Check sheet for the drawn part. Datum: minimum x, y, z corner. Units: mm. Round coordinates to 2 decimals unless told otherwise and drop trailing zeros. Write each loop counter-clockwise with the first axis right and the second up, starting at its lowest first coordinate (ties: lowest second). Pieces come first, ordered by that corner, then holes. Notation, with made-up numbers: M 64.25,39 L 74.25,39 A7 ccw 74.25,51 Z; hole C -28.5,-3 d10. An arc over 180 degrees is marked long. One line per item, written item: value. Start each with the question number.
Item 1: Section check A-A, the plane x = 2.9. Record the cut outline in (y, z).
Item 2: Section check C-C, the plane y = 2.8. Record the cut outline in (x, z).
Item 3: Thickness scan on probe 1 along Z at (x, y) = (2.7, 0.6); probe 2 along Z at (x, y) = (3.2, 2.7); probe 3 along X at (y, z) = (0.45, 1.65) (1 decimal). Record the ranges inside material, lowest first. Write a range as from..to.
Item 4: Draft check along Z on the marked faces 1, 2 and 3. Enter one of: +Z half, -Z half, draft (parallel to the pull), parting line (faces both ways), or undercut.
Item 5: Section check B-B, the plane z = 1.9. Record the cut outline in (x, y).
Item 6: Section check D-D, the plane x = 1. Record the cut outline in (y, z).
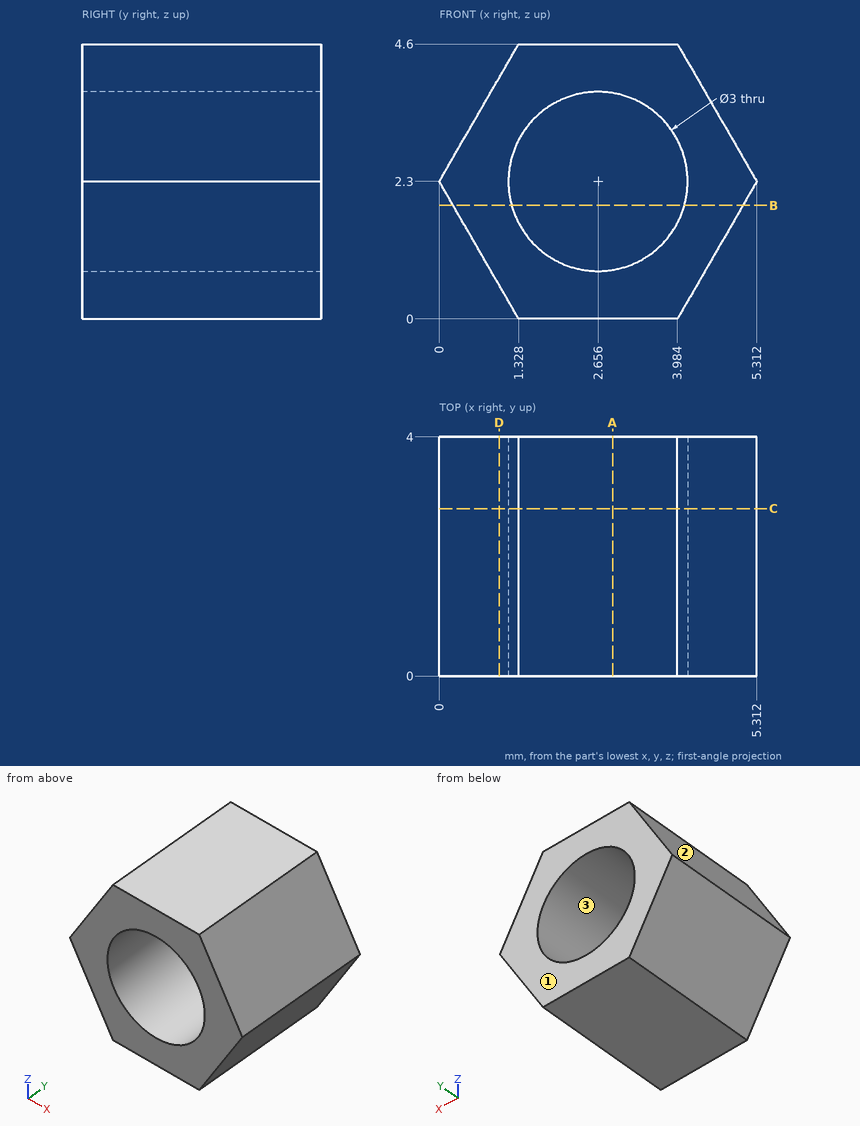
Response values:
1. outline: M 0,0 L 4,0 L 4,0.82 L 0,0.82 Z; M 0,3.78 L 4,3.78 L 4,4.6 L 0,4.6 Z
2. outline: M 0,2.3 L 1.33,0 L 3.98,0 L 5.31,2.3 L 3.98,4.6 L 1.33,4.6 Z; hole C 2.66,2.3 d3
3. probe 1: z = 0..0.8, 3.8..4.6
3. probe 2: z = 0..0.9, 3.7..4.6
3. probe 3: x = 0.4..1.3, 4..4.9
4. face 1: draft
4. face 2: +Z half
4. face 3: undercut
5. outline: M 0.23,0 L 1.21,0 L 1.21,4 L 0.23,4 Z; M 4.1,0 L 5.08,0 L 5.08,4 L 4.1,4 Z
6. outline: M 0,0.57 L 4,0.57 L 4,4.03 L 0,4.03 Z
